from build123d import *

# Parameters (mm, degrees)
F0_W     = 10
F0_H     = 16
F1_DEPTH = 2
F3_DEPTH = 2


# Not quite as in the source:
# - ends of sketch curves that miss each other by under 0.0002 mm in the source are joined


with BuildPart() as f1:
    # F0 (on Top) → F1 (new body)
    with BuildSketch(Plane.XY):
        Rectangle(F0_W, F0_H)
    extrude(amount=F1_DEPTH)

    # F2 (on face) → F3 (join)
    with BuildSketch(Plane.XY.offset(2)):
        Polygon((-2.1414213562, 4.8585786438), (-3.1414213562, 5.8585786438), (-4.1414213562, 4.8585786438), (-4.1414213562, 1.1507223826), (-3.1374518146, 0.1453992321), (-2.1414213562, 1.0335195075), align=None)
        Polygon((2, 0.891659756), (2.00782e-05, 0.9006214721), (-2, 0.891659756), (-3, 0), (-2, -0.891659756), (-2.00782e-05, -0.9006214721), (2, -0.891659756), (3, 0), align=None)
        Polygon((4.1414213562, 4.8585786438), (3.1414213562, 5.8585786438), (2.1414213562, 4.8585786438), (2.1414213562, 1.0335195075), (3.1374518146, 0.1453992321), (4.1414213562, 1.1507223826), align=None)
        Polygon((3.1374518146, -0.1453992321), (2.1414213562, -1.0335195075), (2.1414213562, -4.8585786438), (3.1414213562, -5.8585786438), (4.1414213562, -4.8585786438), (4.1414213562, -1.1507223826), align=None)
    extrude(amount=F3_DEPTH)


solid = f1.part
Check sheet for the modelled part. Datum: model origin and axes. Units: mm. A direction names the side the tool comes from. Round coordinates to 2 decimals unless told otherwise and drop trailing zeros. Order: outer loops, then holes, each group sorted by start corner. A loop starts at its lowest first (then second) coordinate and runs counter-clockwise, first axis right, second up. Notation, with made-up numbers: M 56,-4 L 63,-4 A27 ccw 63,31 Z; hole C 70.5,85.5 d2. An arc over 180 degrees is marked long. One line per item, written item: value. Start each with the question number.
1. Release check for a two-part mould opening along X. For faces 1 (the flat face through (3, 3, 4)), 2 (the flat face through (2.493, -0.452, 2.986)), 3 (the flat face through (2.507, 0.44, 2.986)), 4 (the flat face through (4.141, 3, 3)) record: released by +X, released by -X, zero draft, split by the parting line, or undercut.
2. Gauge pin test, flat ends, axial feed: P1, Ø0.6, axis at y = 2, z = 3, coming from the +X side; P2, Ø1.5, axis at x = 3.5, z = 3, coming from the -Y side; P3, Ø0.6, axis at y = 3, z = 3, coming from the -X side. Record the tip position at first contact, or that the pin passes through.
3. Section check D-D on y = -3.5. Enter the section's corners in (x, z).
4. Scan lines: line 1 along X through (y, z) = (3.5, 2.25); line 2 along Z through (x, y) = (-3, -0.25); line 3 along Y through (x, z) = (0.75, 3.4). Record each from-to range of solid material in increasing order.
5. Access from +Z, -Z, +X, -X, +Y, -Y to the whole of each face (thin tool, end or side, straight path). Record for faces 5 (the flat face through (-2.507, -0.44, 2.986)), 6 (the flat face through (3.63, 0.64, 2.99)), 7 (the flat face through (-2.634, 5.352, 2.986)), 8 (the flat face through (-2.493, 0.452, 2.986)).
6. Section check B-B on y = 2. Enter the section's corners in (x, z), and give its area (3 significant figures).
7. Section check C-C on x = 1.25. Enter the section's corners in (y, z).
8. Section check A-A on z = 2.35. Enter the section's corners in (x, y).
Results found:
1. face 1: zero draft
1. face 2: undercut
1. face 3: undercut
1. face 4: released by +X
2. P1: x = 4.14
2. P2: y = -5.86
2. P3: x = -4.14
3. outline: M -5,0 L 5,0 L 5,2 L 4.14,2 L 4.14,4 L 2.14,4 L 2.14,2 L -5,2 Z
4. line 1: -4.14 to -2.14, 2.14 to 4.14
4. line 2: 0 to 2
4. line 3: -0.9 to 0.9
5. face 5: +Z, -X, -Y
5. face 6: +Z, +X
5. face 7: +Z, +Y
5. face 8: +Z
6. outline: M -5,0 L 5,0 L 5,2 L 4.14,2 L 4.14,4 L 2.14,4 L 2.14,2 L -2.14,2 L -2.14,4 L -4.14,4 L -4.14,2 L -5,2 Z
6. area: 28.0 mm^2
7. outline: M -8,0 L 8,0 L 8,2 L 0.9,2 L 0.9,4 L -0.9,4 L -0.9,2 L -8,2 Z
8. outline: M -4.14,1.15 L -3.14,0.15 L -2.14,1.03 L -2.14,4.86 L -3.14,5.86 L -4.14,4.86 Z; M -3,0 L -2,-0.89 L 0,-0.9 L 2,-0.89 L 3,0 L 2,0.89 L 0,0.9 L -2,0.89 Z; M 2.14,-4.86 L 3.14,-5.86 L 4.14,-4.86 L 4.14,-1.15 L 3.14,-0.15 L 2.14,-1.03 Z; M 2.14,1.03 L 3.14,0.15 L 4.14,1.15 L 4.14,4.86 L 3.14,5.86 L 2.14,4.86 Z
